Can you work these out from the model? Positions are in its coordinate system, mm. A direction names the side the tool comes from. Give positions to 0.01 mm unless a question says otherwise; leave off trailing zeros. Order: outer loops, then holes, each group sorted by start corner. A loop starts at its lowest first (then second) coordinate and runs counter-clockwise, first axis right, second up.
Item 1: I want a section at C-C, the plane z = 5.13. Write out the boundary of the cut face in (x, y).
Item 2: Which directions (+Z, -Z, +X, -X, +Y, -Y) give clear straight access to the entire face, cutting with the end or side of a thin tool? Please do faces 4 (the flat face through (19, 1, 30)), 5 (the flat face through (0, 0, 24)), 6 (the flat face through (-25, 15, 31)).
Item 3: I want a section at A-A, the plane x = 0. Write out the boundary of the cut face in (y, z).
Item 4: I want a section at B-B, the plane y = 5.5. Write out the boundary of the cut face in (x, z), then the cut area to 3 significant figures.
Item 5: If we mould it in two halves opening along X, with no side actions, what happens to faces 1 (the cylindrical face through (-27.859, 25.797, 31.986)), 2 (the flat face through (23, 27, 32)), 3 (the flat face through (-20.5, 12, 32))? For each: +X half, -X half, draft (parallel to the pull), parting line (faces both ways), or undercut.
Item 6: I want a section at D-D, the plane x = 24.25. Write out the boundary of the cut face in (y, z), then the cut area to 3 significant figures.
Item 7: I'm going to push flat-ended pins straight in: pin 1 Ø6.5 at (x, z) = (24.25, 22.13) entering from +Y; pin 2 Ø2 at (x, z) = (-9.75, 32.5) entering from -Y; pin 3 Ø4.5 at (x, y) = (24.25, 9.87) entering from -Z; pin 4 Ø10 at (x, z) = (2.5, 27.5) entering from -Y. Where does each tip first touch, or does it pass through?
Item 8: If I drill on line 1 along Y through (x, z) = (-24.25, 32.4); line 2 along Y through (x, z) = (-24.25, 32.6); line 3 along X through (y, z) = (1.6, 22.13), over which ranges is the centre line in solid material (lowest first)?
```python
from build123d import *

# Parameters (mm, degrees)
T_LE_DE_BASE_PLI_E1_DEPTH             = 20.5
ESQUISSE8_W                           = 24
ESQUISSE8_H                           = 2
BOSS_EXTRU_1_DEPTH                    = 8.5
T_LE_PLI_E_SUR_AR_TE1_STRIP_W         = 10
T_LE_PLI_E_SUR_AR_TE1_STRIP_H         = 2
T_LE_PLI_E_SUR_AR_TE1_STRIP_CUT_DEPTH = 8.5
T_LE_PLI_E_SUR_AR_TE1_DEPTH           = 8.5
ESQUISSE12_W                          = 1.5
ESQUISSE12_H                          = 12
ENL_V_MAT_EXTRU_1_DEPTH               = 8.5
DIAM_TRE_DU_PER_AGE_4_0_4_1_D         = 4
DIAM_TRE_DU_PER_AGE_8_0_8_1_D         = 8
DIAM_TRE_DU_PER_AGE_2_5_2_5_1_D       = 2.5
R_P_TITION_CIRCULAIRE1_COUNT          = 8
DIAM_TRE_DU_PER_AGE_4_0_4_2_D         = 4
DIAM_TRE_DU_PER_AGE_2_5_2_5_2_D       = 2.5
CONG_1_R                              = 4
DIAM_TRE_DU_PER_AGE_8_0_8_2_D         = 8
DIAM_TRE_DU_PER_AGE_2_5_2_5_3_D       = 2.5
R_P_TITION_CIRCULAIRE2_COUNT          = 4


# Sheet-metal steps are written as plain solids
with BuildPart() as part:
    # Esquisse1 → Tôle de base pliée1 (new body)
    with BuildSketch(Plane(origin=(0, 0, 0), x_dir=(0, 0, -1), z_dir=(1, 0, 0))):
        with BuildLine():
            Line((0, 27), (0, 3))
            ThreePointArc((0, 3), (-0.878679656, 0.878679656), (-3, 0))
            Line((-3, 0), (-37.5, 0))
            Line((-37.5, 0), (-37.5, 2))
            Line((-37.5, 2), (-3, 2))
            ThreePointArc((-3, 2), (-2.292893219, 2.292893219), (-2, 3))
            Line((-2, 3), (-2, 27))
            Line((-2, 27), (0, 27))
        make_face()
    extrude(amount=T_LE_DE_BASE_PLI_E1_DEPTH)

    # Esquisse8 → Boss.-Extru.1 (add)
    with BuildSketch(Plane(origin=(20.5, 0, 0), x_dir=(0, 0, -1), z_dir=(1, 0, 0))):
        with Locations((-19, 1)):
            Rectangle(ESQUISSE8_W, ESQUISSE8_H)
    extrude(amount=BOSS_EXTRU_1_DEPTH)

    # Tôle pliée sur arête1 strip (across the edge) → Tôle pliée sur arête1 strip cut (cut)
    with BuildSketch(Plane(origin=(20.5, 2, 31), x_dir=(0, 0, -1), z_dir=(1, 0, 0))):
        with Locations((-4, -1)):
            Rectangle(T_LE_PLI_E_SUR_AR_TE1_STRIP_W, T_LE_PLI_E_SUR_AR_TE1_STRIP_H)
    extrude(amount=T_LE_PLI_E_SUR_AR_TE1_STRIP_CUT_DEPTH, mode=Mode.SUBTRACT)

    # Tôle pliée sur arête1 section (across the edge) → Tôle pliée sur arête1 (add)
    with BuildSketch(Plane(origin=(20.5, 2, 31), x_dir=(0, 0, -1), z_dir=(1, 0, 0))):
        with BuildLine():
            Line((-2, 1), (-2, 25))
            Line((-2, 25), (0, 25))
            Line((0, 25), (0, 1))
            ThreePointArc((0, 1), (0.292893219, 0.292893219), (1, 0))
            Line((1, 0), (1, -2))
            ThreePointArc((1, -2), (-1.121320344, -1.121320344), (-2, 1))
        make_face()
    extrude(amount=T_LE_PLI_E_SUR_AR_TE1_DEPTH)

    # Esquisse12 → Enlèv. mat.-Extru.1 (cut)
    with BuildSketch(Plane(origin=(0, 2, 0), x_dir=(1, 0, 0), z_dir=(0, 1, 0))):
        with Locations((19.75, -31.5)):
            Rectangle(ESQUISSE12_W, ESQUISSE12_H)
    extrude(amount=-ENL_V_MAT_EXTRU_1_DEPTH, mode=Mode.SUBTRACT)

    # Diamètre du perçage Ø4.0 (4)1 (through all)
    with Locations(Plane(origin=(0, 2, 0), x_dir=(1, 0, 0), z_dir=(0, 1, 0))):
        with Locations((24.25, -12.13), (24.25, -22.13)):
            Hole(DIAM_TRE_DU_PER_AGE_4_0_4_1_D / 2)

    # Diamètre du perçage Ø8.0 (8)1 (through all)
    with Locations(Plane(origin=(0, 2, 0), x_dir=(1, 0, 0), z_dir=(0, 1, 0))):
        with Locations((9.75, -25.5)):
            Hole(DIAM_TRE_DU_PER_AGE_8_0_8_1_D / 2)

    # Diamètre du perçage Ø2.5 (2.5)1 (through all)
    with Locations(Plane(origin=(0, 2, 0), x_dir=(1, 0, 0), z_dir=(0, 1, 0))):
        with Locations((9.75, -18.5)):
            diam_tre_du_per_age_2_5_2_5_1 = Hole(DIAM_TRE_DU_PER_AGE_2_5_2_5_1_D / 2)

    # Répétition circulaire1: Diamètre du perçage Ø2.5 (2.5)1 ×8 about axis, 3 skipped
    r_p_tition_circulaire1_axis = Axis((9.75, 2, 25.5), (0, 1, 0))
    add([diam_tre_du_per_age_2_5_2_5_1.rotate(r_p_tition_circulaire1_axis, i * 360 / R_P_TITION_CIRCULAIRE1_COUNT) for i in range(1, R_P_TITION_CIRCULAIRE1_COUNT) if i not in (1, 3, 6)], mode=Mode.SUBTRACT)

    # Diamètre du perçage Ø4.0 (4)2 (through all)
    with Locations(Plane.XY.offset(33)):
        with Locations((24.25, 19.87), (24.25, 9.87)):
            Hole(DIAM_TRE_DU_PER_AGE_4_0_4_2_D / 2)

    # Diamètre du perçage Ø2.5 (2.5)2 (through all)
    with Locations(Plane.XY.offset(2)):
        with Locations((10, 14.87)):
            Hole(DIAM_TRE_DU_PER_AGE_2_5_2_5_2_D / 2)

    # Congé1
    cong_1_edges = [part.edges().sort_by_distance(p)[0] for p in [
        (20.5, 27, 1),
        (29, 1, 7),
        (29, 27, 32),
        (19, 1, 37.5),
    ]]
    fillet(cong_1_edges, radius=CONG_1_R)

    # Symétrie1: part across plane


with BuildPart() as part_1:
    add(part.part)
    add(part.part.mirror(Plane(origin=(0, 3, 3), x_dir=(0, 0, 1), z_dir=(1, 0, 0))))

    # Diamètre du perçage Ø8.0 (8)2 (through all)
    with Locations(Plane(origin=(0, 2, 0), x_dir=(1, 0, 0), z_dir=(0, 1, 0))):
        with Locations((0, -12.13)):
            Hole(DIAM_TRE_DU_PER_AGE_8_0_8_2_D / 2)

    # Diamètre du perçage Ø2.5 (2.5)3 (through all)
    with Locations(Plane(origin=(0, 2, 0), x_dir=(1, 0, 0), z_dir=(0, 1, 0))):
        with Locations((0, -5.13)):
            diam_tre_du_per_age_2_5_2_5_3 = Hole(DIAM_TRE_DU_PER_AGE_2_5_2_5_3_D / 2)

    # Répétition circulaire2: Diamètre du perçage Ø2.5 (2.5)3 ×4 about axis
    r_p_tition_circulaire2_axis = Axis((0, 0, 12.13), (0, 1, 0))
    for i in range(1, R_P_TITION_CIRCULAIRE2_COUNT):
        add(diam_tre_du_per_age_2_5_2_5_3.rotate(r_p_tition_circulaire2_axis, i * 360 / R_P_TITION_CIRCULAIRE2_COUNT), mode=Mode.SUBTRACT)


solid = part_1.part
```
Results list:
1. outline: (-20.5, 0) - (-1.25, 0) - (-1.25, 2) - (-20.5, 2) - close; (1.25, 0) - (20.5, 0) - (20.5, 2) - (1.25, 2) - close
2. face 4: +Z, +Y, -Y
2. face 5: +Z, -Z, +X, -X, -Y
2. face 6: -Z, +X, -X, +Y
3. outline: (0, 3) arc R3 ccw to (3, 0) - (27, 0) - (27, 2) - (3, 2) arc R1 cw to (2, 3) - (2, 3.88) - (0, 3.88) - close; (0, 6.38) - (2, 6.38) - (2, 8.13) - (0, 8.13) - close; (0, 16.13) - (2, 16.13) - (2, 17.88) - (0, 17.88) - close; (0, 20.38) - (2, 20.38) - (2, 37.5) - (0, 37.5) - close
4. outline: (-29, 31) - (-20.5, 31) - (-20.5, 33) - (-29, 33) - close; (-20.5, 0) - (20.5, 0) - (20.5, 2) - (-20.5, 2) - close; (20.5, 31) - (29, 31) - (29, 33) - (20.5, 33) - close
4. area: 116 mm2
5. face 1: -X half
5. face 2: draft
5. face 3: undercut
6. outline: (0, 7) - (2, 7) - (2, 10.13) - (0, 10.13) - close; (0, 14.13) - (2, 14.13) - (2, 20.13) - (0, 20.13) - close; (0, 24.13) - (2, 24.13) - (2, 30) arc R1 cw to (3, 31) - (7.87, 31) - (7.87, 33) - (3, 33) arc R3 ccw to (0, 30) - close; (11.87, 31) - (17.87, 31) - (17.87, 33) - (11.87, 33) - close; (21.87, 31) - (27, 31) - (27, 33) - (21.87, 33) - close
6. area: 68.3 mm2
7. pin 1: stops at y = 2
7. pin 2: passes through
7. pin 3: stops at z = 31
7. pin 4: stops at y = 0
8. line 1: y = 1.2 to 7.87, 11.87 to 17.87, 21.87 to 27
8. line 2: y = 1.5 to 7.87, 11.87 to 17.87, 21.87 to 27
8. line 3: x = -29 to -26.25, -22.25 to -11.9, -7.6 to 7.6, 11.9 to 22.25, 26.25 to 29
